from build123d import *

# Parameters (mm, degrees)
SKETCH1_W           = 74.5
SKETCH1_H           = 70
BOSS_EXTRUDE1_DEPTH = 18
SKETCH3_W           = 5
SKETCH3_H           = 10
SKETCH3_W_2         = 8.5
SKETCH3_H_2         = 5
SKETCH3_W_3         = 18.5
SKETCH3_W_4         = 16.5
SKETCH3_H_3         = 15
CUT_EXTRUDE1_DEPTH  = 5
SKETCH4_W           = 45
SKETCH4_H           = 12
SKETCH4_R           = 2.5
BOSS_EXTRUDE2_DEPTH = 2.5
SKETCH5_W           = 15
SKETCH5_H           = 18
SKETCH5_R           = 2.5
BOSS_EXTRUDE3_DEPTH = 2.5
SKETCH6_R           = 2
CUT_EXTRUDE2_DEPTH  = 19


with BuildPart() as part:
    # Sketch1 → Boss-Extrude1 (new body)
    with BuildSketch(Plane(origin=(0, 0, 0), x_dir=(1, 0, 0), z_dir=(0, 1, 0))):
        Rectangle(SKETCH1_W, SKETCH1_H)
    extrude(amount=BOSS_EXTRUDE1_DEPTH)

    # Sketch3 → Cut-Extrude1 (cut)
    with BuildSketch(Plane(origin=(0, 18, 0), x_dir=(1, 0, 0), z_dir=(0, 1, 0))):
        with Locations((-24.75, -26.5)):
            Rectangle(SKETCH3_W, SKETCH3_H)
        with Locations((-18, -29)):
            Rectangle(SKETCH3_W_2, SKETCH3_H_2)
        Polygon((-28.75, -21.5), (-27.25, -21.5), (-22.25, -21.5), (-20.75, -21.5), (-20.75, -19.8), (-22.25, -18.3), (-27.25, -18.3), (-28.75, -19.8), align=None)
        with Locations((0.5, -29)):
            Rectangle(SKETCH3_W_3, SKETCH3_H_2)
        with Locations((18, -29)):
            Rectangle(SKETCH3_W_4, SKETCH3_H_2)
        with Locations((27.25, -14.5)):
            Rectangle(SKETCH3_W, SKETCH3_H_3)
    extrude(amount=-CUT_EXTRUDE1_DEPTH, mode=Mode.SUBTRACT)

    # Sketch4 → Boss-Extrude2 (add)
    with BuildSketch(Plane(origin=(37.25, 0, 0), x_dir=(0, 0, -1), z_dir=(1, 0, 0))):
        with Locations((12.5, 12)):
            Rectangle(SKETCH4_W, SKETCH4_H)
        with Locations((25, 12)):
            Circle(SKETCH4_R, mode=Mode.SUBTRACT)
        with Locations((12.5, 12)):
            Circle(SKETCH4_R, mode=Mode.SUBTRACT)
        with Locations((0, 12)):
            Circle(SKETCH4_R, mode=Mode.SUBTRACT)
    extrude(amount=BOSS_EXTRUDE2_DEPTH)

    # Sketch5 → Boss-Extrude3 (add)
    with BuildSketch(Plane.ZY.offset(37.25)):
        with Locations((-17, 9)):
            Rectangle(SKETCH5_W, SKETCH5_H)
        with Locations((-17, 12)):
            Circle(SKETCH5_R, mode=Mode.SUBTRACT)
        with Locations((-17, 6)):
            Circle(SKETCH5_R, mode=Mode.SUBTRACT)
    extrude(amount=BOSS_EXTRUDE3_DEPTH)

    # Sketch6 → Cut-Extrude2 (cut, through all)
    with BuildSketch(Plane.XZ):
        with Locations((-33.75, 21)):
            Circle(SKETCH6_R)
        with Locations((-33.75, -18)):
            Circle(SKETCH6_R)
    cut_extrude2 = extrude(amount=-CUT_EXTRUDE2_DEPTH, mode=Mode.SUBTRACT)

    # Mirror1: Cut-Extrude2 across plane
    add(cut_extrude2.mirror(Plane(origin=(0, 0, 0), x_dir=(0, 0, 1), z_dir=(1, 0, 0))), mode=Mode.SUBTRACT)


solid = part.part
The model under review builds one solid part; all positions refer to its coordinate system, in mm. A direction names the side the tool comes from. Give positions to 0.01 mm unless a question says otherwise; leave off trailing zeros. Write each loop counter-clockwise with the first axis right and the second up, starting at its lowest first coordinate (ties: lowest second). Pieces come first, ordered by that corner, then holes.
1. Add section B-B, the plane y = 12. Count the separate pieces of the cut face and the enclosed holes in it, plus the area to 3 significant figures.
2. Add section C-C, the plane z = -17. Write out the cut boundary in (x, y).
3. For P1, Ø3, axis at y = 12, z = -12.5, coming from the +X side; P2, Ø6, axis at x = -28, z = 26.5, coming from the -Y side; P3, Ø5, axis at y = 11.5, z = 21, coming from the -X side; P4, Ø0.8, axis at x = -39, y = 8.5, coming from the -Z side, all flat-tipped, find the tip position at first contact; note any pin that passes through.
4. Add section A-A, the plane x = 33.75. Write out the cut boundary in (y, z).
5. Tool access review of faces 5 (the flat face through (39.75, 9, -12)), 6 (the flat face through (27, 16, 22)), 7 (the cylindrical face through (38.48, 9.56, 0.54)), 8 (the flat face through (-2, 0, 0)), 9 (the flat face through (-37.25, 12, -17)): name each direction out of +Z, -Z, +X, -X, +Y, -Y from which nothing blocks a thin tool from reaching the whole face with its end or side.
6. Add section D-D, the plane z = 15. Write out the cut boundary in (x, y), plus the area to 3 significant figures.
7. Wall thickness on L1, parallel to Z at x = 33.75, y = 9; L2, parallel to Y at x = -38, z = -17; L3, parallel to X at y = 2.25, z = 20: over which ranges is each line inside the solid? List them lowest first.
8. Draft analysis for pull direction Z (two halves, no side actions). For faces 1 (the flat face through (9, 13, 29)), 2 (the flat face through (-1, 18, 0)), 3 (the flat face through (38, 12, 10)), 4 (the flat face through (1, 9, -35)), state which applies: +Z half, -Z half, draft (parallel to the pull), parting line (faces both ways), or undercut.
Worked answers:
1. separate pieces: 1
1. enclosed holes: 4
1. area: 5,260 mm2
2. outline: (-39.75, 0) - (-35.48, 0) - (-35.48, 18) - (-39.75, 18) - (-39.75, 14.5) - (-37.25, 14.5) - (-37.25, 9.5) - (-39.75, 9.5) - (-39.75, 8.5) - (-37.25, 8.5) - (-37.25, 3.5) - (-39.75, 3.5) - close; (-32.02, 0) - (32.02, 0) - (32.02, 18) - (-32.02, 18) - close; (35.48, 0) - (37.25, 0) - (37.25, 6) - (39.75, 6) - (39.75, 18) - (35.48, 18) - close
3. P1: stops at x = 37.25
3. P2: stops at y = 0
3. P3: stops at x = -37.25
3. P4: stops at z = -24.5
4. outline: (0, -35) - (18, -35) - (18, -20) - (0, -20) - close; (0, -16) - (18, -16) - (18, 19) - (0, 19) - close; (0, 23) - (18, 23) - (18, 35) - (0, 35) - close
5. face 5: +Z, -Z, +X, +Y, -Y
5. face 6: +Y
5. face 7: +X
5. face 8: +Z, -Z, +X, -X, -Y
5. face 9: -X
6. outline: (-37.25, 0) - (37.25, 0) - (37.25, 18) - (29.75, 18) - (29.75, 13) - (24.75, 13) - (24.75, 18) - (-37.25, 18) - close
6. area: 1,320 mm2
7. L1: z = -35 to -20, -16 to 19, 23 to 35
7. L2: y = 0 to 3.5, 8.5 to 9.5, 14.5 to 18
7. L3: x = -37.25 to -35.48, -32.02 to 32.02, 35.48 to 37.25
8. face 1: undercut
8. face 2: draft
8. face 3: +Z half
8. face 4: -Z half
